Geometry: see drawing. Coordinates: mm, zero at the bounding-box minimum. A direction names the side the tool comes from. Coordinates: 2 decimals unless noted, no trailing zeros. Loops run counter-clockwise (first coordinate to the right, second up) from the corner with the lowest first, then second, coordinate; pieces in that order, holes last. Notation, with made-up numbers: (67.25, 63) -> (91.25, 63) arc R9 ccw to (91.25, 69) -> close; hole circle Ø5 at (64, 76). An arc over 180 degrees is marked (long way). Answer as a JSON object with one key per item and string values.
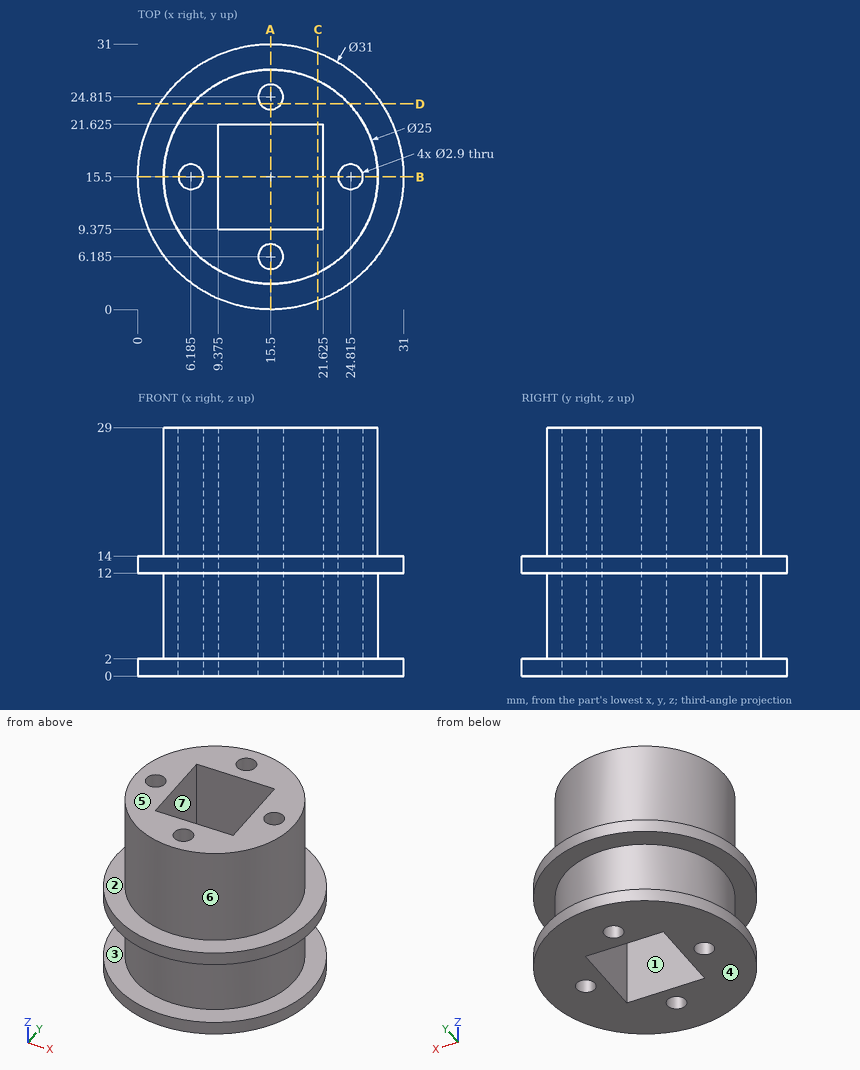
1. Section query A-A (x = 15.5). Return loops of the section in (y, z) (3 decimals).
Reply:
{"outline": "(0, 0) -> (4.735, 0) -> (4.735, 29) -> (3, 29) -> (3, 14) -> (0, 14) -> (0, 12) -> (3, 12) -> (3, 2) -> (0, 2) -> close; (7.635, 0) -> (9.375, 0) -> (9.375, 29) -> (7.635, 29) -> close; (21.625, 0) -> (23.365, 0) -> (23.365, 29) -> (21.625, 29) -> close; (26.265, 0) -> (31, 0) -> (31, 2) -> (28, 2) -> (28, 12) -> (31, 12) -> (31, 14) -> (28, 14) -> (28, 29) -> (26.265, 29) -> close"}
2. Mould query, pull axis X, two halves, no side actions, for the marked faces 5, 6 and 7. Classes: pulls with the +X half, pulls with the -X half, needs draft (parallel to the pull), parting line crosses it, or undercut.
Reply:
{"face 5": "needs draft", "face 6": "parting line crosses it", "face 7": "undercut"}
3. Line query: line 1 along Y through (x, z) = (15.5, 15) (3 decimals); line 2 along Z through (x, y) = (2.5, 11); line 3 along Y through (x, z) = (16, 26.5) (3 decimals). Output: solid intervals per line, ascending.
Reply:
{"line 1": "y = 3 to 4.735, 7.635 to 9.375, 21.625 to 23.365, 26.265 to 28", "line 2": "z = 0 to 2, 12 to 14", "line 3": "y = 3.01 to 4.824, 7.546 to 9.375, 21.625 to 23.454, 26.176 to 27.99"}
4. Section query D-D (y = 24). Return loops of the section in (x, z).
Reply:
{"outline": "(2.54, 0) -> (14.3, 0) -> (14.3, 29) -> (6.33, 29) -> (6.33, 14) -> (2.54, 14) -> (2.54, 12) -> (6.33, 12) -> (6.33, 2) -> (2.54, 2) -> close; (16.7, 0) -> (28.46, 0) -> (28.46, 2) -> (24.67, 2) -> (24.67, 12) -> (28.46, 12) -> (28.46, 14) -> (24.67, 14) -> (24.67, 29) -> (16.7, 29) -> close"}
5. Pin query (flat end, axial travel): P1, Ø2, axis at y = 25.5, z = 22, coming from the -X side; P2, Ø3, axis at y = 4, z = 7.5, coming from the +X side; P3, Ø1.7, axis at x = 15.5, y = 24.815, coming from the -Z side; P4, Ø6, axis at x = 28, z = 8.5, coming from the -Y side. Return the tip coordinate at first contact, or that it passes through.
Reply:
{"P1": "stops at x = 6.83", "P2": "stops at x = 23", "P3": "passes through", "P4": "stops at y = 7.38"}
6. Section query C-C (x = 21). Return loops of the section in (y, z) (3 decimals).
Reply:
{"outline": "(1.009, 0) -> (9.375, 0) -> (9.375, 29) -> (4.275, 29) -> (4.275, 14) -> (1.009, 14) -> (1.009, 12) -> (4.275, 12) -> (4.275, 2) -> (1.009, 2) -> close; (21.625, 0) -> (29.991, 0) -> (29.991, 2) -> (26.725, 2) -> (26.725, 12) -> (29.991, 12) -> (29.991, 14) -> (26.725, 14) -> (26.725, 29) -> (21.625, 29) -> close"}
7. Access query for the marked faces 1, 2, 3 and 4. Directions: +Z, -Z, +X, -X, +Y, -Y. A direction counts if a zero-diameter tool reaches every point of the face in a straight line with its end or side. Return the directions, or none.
Reply:
{"face 1": "+Z, -Z", "face 2": "+Z", "face 3": "none", "face 4": "-Z, +X, -X, +Y, -Y"}
